```python
from build123d import *

# Parameters (mm, degrees)
F0_W     = 31.75
F0_H     = 50.8
F1_DEPTH = 482.6
F3_DEPTH = 19.05
F5_DEPTH = 19.05


with BuildPart() as f1:
    # F0 (on Front) → F1 (new body)
    with BuildSketch(Plane.XZ):
        Rectangle(F0_W, F0_H)
    extrude(amount=F1_DEPTH)

    # F2 (on face) → F3 (join)
    with BuildSketch(Plane(origin=(0, 0, 0), x_dir=(-1, 0, 0), z_dir=(0, 1, 0))):
        with BuildLine():
            Line((-6.35, 6.35), (-6.35, -6.35))
            ThreePointArc((-6.35, -6.35), (0, -12.7), (6.35, -6.35))
            Line((6.35, -6.35), (6.35, 6.35))
            ThreePointArc((6.35, 6.35), (0, 12.7), (-6.35, 6.35))
        make_face()
    extrude(amount=F3_DEPTH)

    # F4 (on face) → F5 (join)
    with BuildSketch(Plane.XZ.offset(482.6)):
        with BuildLine():
            Line((-6.35, 6.35), (-6.35, -6.35))
            ThreePointArc((-6.35, -6.35), (0, -12.7), (6.35, -6.35))
            Line((6.35, -6.35), (6.35, 6.35))
            ThreePointArc((6.35, 6.35), (0, 12.7), (-6.35, 6.35))
        make_face()
    extrude(amount=F5_DEPTH)


solid = f1.part
```
Here's how the part is built. I have some questions about the finished solid (model axes, mm). A direction names the side the tool comes from. Round coordinates to 2 decimals unless told otherwise and drop trailing zeros. Write each loop counter-clockwise with the first axis right and the second up, starting at its lowest first coordinate (ties: lowest second). Pieces come first, ordered by that corner, then holes. Notation, with made-up numbers: M 55.5,9 L 94.5,9 A28 cw 94.5,33 Z; hole C 82.5,66.25 d11. An arc over 180 degrees is marked long. Answer as CSV lines item,"result". Start each with the question number.
1. Suppose I cut it at A-A on x = 0. Write out the boundary of the cut face in (y, z).
2. I need wall thicknesses on probe 1 along Y at (x, z) = (-13, 10). Which ranges of the line are inside material? Lowest first, please.
3. On a 3-axis mill with a long thin cutter (end or side, diameter ignored), from which of +Z, -Z, +X, -X, +Y, -Y can I reach the whole of each face in a straight line? I mean faces 1 (the cylindrical face through (0.1, -492, 12.7)), 2 (the cylindrical face through (-0.1, 9.4, 12.7)), 3 (the flat face through (6.35, 9, 0)), 4 (the flat face through (-6.35, -492, 0)). Say none if no direction works.
4. I'm going to push flat-ended pins straight in: pin 1 Ø5 at (x, z) = (-5.5, -11.5) entering from -Y; pin 2 Ø14 at (y, z) = (11, -3) entering from -X; pin 3 Ø8 at (x, z) = (12, -6) entering from +Y. Where does each tip first touch, or does it pass through?
Check result:
1,outline,"M -501.65,-12.7 L -482.6,-12.7 L -482.6,-25.4 L 0,-25.4 L 0,-12.7 L 19.05,-12.7 L 19.05,12.7 L 0,12.7 L 0,25.4 L -482.6,25.4 L -482.6,12.7 L -501.65,12.7 Z"
2,probe 1,"y = -482.6 to 0"
3,face 1,"+Z, -Y"
3,face 2,"+Z, +Y"
3,face 3,"+Z, -Z, +X, +Y"
3,face 4,"+Z, -Z, -X, -Y"
4,pin 1,"stops at y = -501.65"
4,pin 2,"stops at x = -6.35"
4,pin 3,"stops at y = 0"
